from build123d import *

# Parameters (mm, degrees)
EXTRUDE_THIN1_DEPTH = 10
FILLET1_R           = 4
SKETCH2_W           = 5
SKETCH2_H           = 12
BOSS_EXTRUDE1_DEPTH = 9.5
SKETCH3_W           = 32.8
SKETCH3_H           = 12
BOSS_EXTRUDE2_DEPTH = 3
FILLET2_R           = 4
SKETCH4_R           = 1.3
CUT_EXTRUDE1_DEPTH  = 3
SKETCH5_R           = 1.5
CUT_EXTRUDE2_DEPTH  = 6
SKETCH6_W           = 32.8
SKETCH6_H           = 10
BOSS_EXTRUDE3_DEPTH = 5
FILLET3_R           = 4
FILLET4_R           = 4
SKETCH7_R           = 2.75
CUT_EXTRUDE3_DEPTH  = 1.5
SKETCH9_W           = 9
SKETCH9_H           = 14
BOSS_EXTRUDE5_DEPTH = 5
FILLET10_R          = 1
SKETCH12_W          = 33
SKETCH12_H          = 14
BOSS_EXTRUDE7_DEPTH = 3
SKETCH13_W          = 5.2
SKETCH13_H          = 14
BOSS_EXTRUDE8_DEPTH = 12.5
FILLET11_R          = 2
FILLET13_R          = 2
SKETCH14_R          = 1.6
CUT_EXTRUDE4_DEPTH  = 58.189247273


with BuildPart() as part:
    # Sketch1 → Extrude-Thin1 (new body)
    with BuildSketch(Plane.XY):
        Polygon((-11.4, -12), (-11.4, 0), (11.4, 0), (11.4, -12), (16.4, -12), (16.4, 5), (-16.4, 5), (-16.4, -12), align=None)
    extrude(amount=EXTRUDE_THIN1_DEPTH)

    # Fillet1
    fillet1_edges = [part.edges().sort_by_distance(p)[0] for p in [
        (-16.4, 5, 5),
        (16.4, 5, 5),
    ]]
    fillet(fillet1_edges, radius=FILLET1_R)

    # Sketch2 → Boss-Extrude1 (add)
    with BuildSketch(Plane.XY.offset(10)):
        with Locations((-13.9, -6)):
            Rectangle(SKETCH2_W, SKETCH2_H)
        with Locations((13.9, -6)):
            Rectangle(SKETCH2_W, SKETCH2_H)
    extrude(amount=BOSS_EXTRUDE1_DEPTH)

    # Sketch3 → Boss-Extrude2 (add)
    with BuildSketch(Plane.XY.offset(19.5)):
        with Locations((0, -6)):
            Rectangle(SKETCH3_W, SKETCH3_H)
    extrude(amount=BOSS_EXTRUDE2_DEPTH)

    # Fillet2
    fillet2_edges = [part.edges().sort_by_distance(p)[0] for p in [
        (13.9, 0, 10),
        (-13.9, 0, 10),
        (16.4, -6, 22.5),
        (-16.4, -6, 22.5),
    ]]
    fillet(fillet2_edges, radius=FILLET2_R)

    # Sketch4 → Cut-Extrude1 (cut)
    with BuildSketch(Plane(origin=(0, 0, 19.5), x_dir=(-1, 0, 0), z_dir=(0, 0, -1))):
        with Locations((5.35, -6.05)):
            Circle(SKETCH4_R)
    extrude(amount=-CUT_EXTRUDE1_DEPTH, mode=Mode.SUBTRACT)

    # Sketch5 → Cut-Extrude2 (cut)
    with BuildSketch(Plane(origin=(0, 0, 0), x_dir=(-1, 0, 0), z_dir=(0, 0, -1))):
        with Locations((14.3, -6.05)):
            Circle(SKETCH5_R)
        with Locations((-14.1, -6.05)):
            Circle(SKETCH5_R)
    extrude(amount=-CUT_EXTRUDE2_DEPTH, mode=Mode.SUBTRACT)

    # Sketch6 → Boss-Extrude3 (add)
    with BuildSketch(Plane.XZ.offset(12)):
        with Locations((0, 5)):
            Rectangle(SKETCH6_W, SKETCH6_H)
    extrude(amount=BOSS_EXTRUDE3_DEPTH)

    # Fillet3
    fillet3_edges = [part.edges().sort_by_distance(p)[0] for p in [
        (16.4, -17, 5),
        (-16.4, -17, 5),
    ]]
    fillet(fillet3_edges, radius=FILLET3_R)

    # Fillet4
    fillet4_edges = [part.edges().sort_by_distance(p)[0] for p in [
        (13.9, -12, 10),
        (-13.9, -12, 10),
    ]]
    fillet(fillet4_edges, radius=FILLET4_R)

    # Sketch7 → Cut-Extrude3 (cut)
    with BuildSketch(Plane(origin=(0, 0, 19.5), x_dir=(-1, 0, 0), z_dir=(0, 0, -1))):
        with Locations((5.35, -6.05)):
            Circle(SKETCH7_R)
    extrude(amount=-CUT_EXTRUDE3_DEPTH, mode=Mode.SUBTRACT)

    # Sketch9 → Boss-Extrude5 (add)
    with BuildSketch(Plane(origin=(16.4, 0, 0), x_dir=(0, 0, -1), z_dir=(1, 0, 0))):
        with Locations((-7.5, -6)):
            Rectangle(SKETCH9_W, SKETCH9_H)
    extrude(amount=BOSS_EXTRUDE5_DEPTH)

    # Fillet10
    fillet10_edges = [part.edges().sort_by_distance(p)[0] for p in [
        (16.4, -6, 12),
    ]]
    fillet(fillet10_edges, radius=FILLET10_R)

    # Sketch12 → Boss-Extrude7 (add)
    with BuildSketch(Plane(origin=(0, 0, 0), x_dir=(-1, 0, 0), z_dir=(0, 0, -1))):
        with Locations((-32.9, -6)):
            Rectangle(SKETCH12_W, SKETCH12_H)
    extrude(amount=-BOSS_EXTRUDE7_DEPTH)

    # Sketch13 → Boss-Extrude8 (add)
    with BuildSketch(Plane.XY.offset(3)):
        with Locations((46.8, -6)):
            Rectangle(SKETCH13_W, SKETCH13_H)
    extrude(amount=BOSS_EXTRUDE8_DEPTH)

    # Fillet11
    fillet11_edges = [part.edges().sort_by_distance(p)[0] for p in [
        (21.4, -6, 12),
    ]]
    fillet(fillet11_edges, radius=FILLET11_R)

    # Fillet13
    fillet13_edges = [part.edges().sort_by_distance(p)[0] for p in [
        (49.4, -6, 15.5),
        (44.2, -6, 15.5),
    ]]
    fillet(fillet13_edges, radius=FILLET13_R)

    # Sketch14 → Cut-Extrude4 (cut, through all)
    with BuildSketch(Plane(origin=(0, 1, 0), x_dir=(1, 0, 0), z_dir=(0, 1, 0))):
        with Locations(Location((18.7, -9.05, 0), (0, 0, 180))):
            Circle(SKETCH14_R)
        with Locations(Location((47.1, -9.05, 0), (0, 0, 180))):
            Circle(SKETCH14_R)
    extrude(amount=-CUT_EXTRUDE4_DEPTH, mode=Mode.SUBTRACT)


solid = part.part
Read the model definition and answer for the solid it produces. Units are mm, in the model's axes. A direction names the side the tool comes from. Give positions to 0.01 mm unless a question says otherwise; leave off trailing zeros. Loops run counter-clockwise (first coordinate to the right, second up) from the corner with the lowest first, then second, coordinate; pieces in that order, holes last. Notation, with made-up numbers: (-14.75, -39) -> (36.25, -39) arc R21 cw to (36.25, -27) -> close; hole circle Ø3 at (14.5, 74). An arc over 180 degrees is marked (long way). Use a Markdown table: item, result.
Q1. Each of these flat-tipped pins is pushed along its axis until it touches: pin 1 (4 mm diameter, centred on x = -0.5, y = 3.5, fed in from +Z); pin 2 (12 mm diameter, centred on x = 25, z = 14.5, fed in from -Y); pin 3 (2.5 mm diameter, centred on x = 18.5, y = -2.5, fed in from +Z); pin 4 (2 mm diameter, centred on x = -5.35, y = -6.05, fed in from -Z). Where does it stop, or does it pass through?
Solved:
| item | result |
|---|---|
| pin 1 | stops at z = 10 |
| pin 2 | stops at y = -13 |
| pin 3 | stops at z = 12.01 |
| pin 4 | passes through |
Q2. A tool of negligible diameter and unlimited length cuts with its end or side. For faces 4 (the face through (20.8, -5.9, 11.43)), 5 (the face through (-13.865, -13.203, 11.141)), 6 (the face through (0, -6, 19.5)), 7 (the face through (47, -6, 15.5)), 8 (the face through (-14, -6, 6)), from which of +Z, -Z, +X, -X, +Y, -Y can it reach the whole face along a straight path? Write none if from no direction.
Solved:
| item | result |
|---|---|
| face 4 | +Z, +Y, -Y |
| face 5 | +Z, -X, -Y |
| face 6 | -Z, +Y, -Y |
| face 7 | +Z, +X, +Y, -Y |
| face 8 | -Z |
Q3. Section A-A, the plane z = 9.05 is taken. Determine the outline of the cut face in (x, y), then the cut area to 3 significant figures.
Solved:
| item | result |
|---|---|
| outline | (-16.4, -13) arc R4 ccw to (-12.4, -17) -> (12.4, -17) arc R4 ccw to (16.4, -13) -> (17.1, -13) -> (17.1, 1) -> (16.4, 1) arc R4 ccw to (12.4, 5) -> (-12.4, 5) arc R4 ccw to (-16.4, 1) -> close; (20.3, -13) -> (21.4, -13) -> (21.4, 1) -> (20.3, 1) -> close; (44.2, -13) -> (45.5, -13) -> (45.5, 1) -> (44.2, 1) -> close; (48.7, -13) -> (49.4, -13) -> (49.4, 1) -> (48.7, 1) -> close; hole (-11.4, -12) -> (11.4, -12) -> (11.4, 0) -> (-11.4, 0) -> close |
| area | 487 mm^2 |
Q4. Determine the mould class of faces 1 (the face through (16.4, -6, 16)), 2 (the face through (0, -17, 5)), 3 (the face through (-15.197, 3.859, 5.757)) for opening direction X: pulls with the +X half, pulls with the -X half, needs draft (parallel to the pull), parting line crosses it, or undercut.
Solved:
| item | result |
|---|---|
| face 1 | undercut |
| face 2 | needs draft |
| face 3 | pulls with the -X half |
Q5. Section D-D, the plane z = 1.5 is taken. Determine the outline of the cut face in (x, y), then the cut area to 3 significant figures.
Solved:
| item | result |
|---|---|
| outline | (-16.4, -13) arc R4 ccw to (-12.4, -17) -> (12.4, -17) arc R4 ccw to (16.4, -13) -> (49.4, -13) -> (49.4, 1) -> (16.4, 1) arc R4 ccw to (12.4, 5) -> (-12.4, 5) arc R4 ccw to (-16.4, 1) -> close; hole circle Ø3 at (-14.3, -6.05); hole (-11.4, -12) -> (11.4, -12) -> (11.4, 0) -> (-11.4, 0) -> close; hole circle Ø3 at (14.1, -6.05) |
| area | 882 mm^2 |
Q6. Find the intervals of material crossed by line 1 along X through (y, z) = (-4.75, 7); line 2 along Y through (x, z) = (7, 4.5); line 3 along X through (y, z) = (-8.5, 17.5), in increasing order.
Solved:
| item | result |
|---|---|
| line 1 | x = -16.4 to -11.4, 11.4 to 21.4, 44.2 to 49.4 |
| line 2 | y = -17 to -12, 0 to 5 |
| line 3 | x = -16.4 to -11.4, 11.4 to 16.4 |
Q7. Section C-C, the plane y = -1.5 is taken. Determine the outline of the cut face in (x, z), then the cut area to 3 significant figures.
Solved:
| item | result |
|---|---|
| outline | (-16.4, 0) -> (-11.4, 0) -> (-11.4, 19.5) -> (11.4, 19.5) -> (11.4, 0) -> (49.4, 0) -> (49.4, 13.5) arc R2 ccw to (47.4, 15.5) -> (46.2, 15.5) arc R2 ccw to (44.2, 13.5) -> (44.2, 3) -> (21.4, 3) -> (21.4, 10) arc R2 ccw to (19.4, 12) -> (17.4, 12) arc R1 cw to (16.4, 13) -> (16.4, 18.5) arc R4 ccw to (12.4, 22.5) -> (-12.4, 22.5) arc R4 ccw to (-16.4, 18.5) -> close; hole circle Ø3.2 at (18.7, 9.05); hole circle Ø3.2 at (47.1, 9.05) |
| area | 477 mm^2 |
Q8. Section B-B, the plane x = 5 is taken. Determine the outline of the cut face in (y, z), then the cut area to 3 significant figures.
Solved:
| item | result |
|---|---|
| outline | (-17, 0) -> (-12, 0) -> (-12, 10) -> (-17, 10) -> close; (-12, 19.5) -> (0, 19.5) -> (0, 22.5) -> (-12, 22.5) -> close; (0, 0) -> (5, 0) -> (5, 10) -> (0, 10) -> close |
| area | 136 mm^2 |
